```python
from build123d import *

# Parameters (mm, degrees)
BOSS_EXTRUDE1_DEPTH      = 6
BOSS_EXTRUDE2_DEPTH      = 40
CUT_EXTRUDE1_REACH       = 62.762
SKETCH9_R                = 1.6
CUT_EXTRUDE2_REACH       = 62.762
SKETCH10_R               = 7
BOSS_EXTRUDE4_DEPTH      = 25
BOSS_EXTRUDE5_REACH      = 73.576
SKETCH12_R               = 2.5
BOSS_EXTRUDE6_REACH      = 73.576
BOSS_EXTRUDE6_END_RADIUS = 23.21251372
SKETCH14_R               = 2.5
SKETCH17_W               = 26.966711831
SKETCH17_H               = 26.757667553
CUT_EXTRUDE4_DEPTH       = 6
FILLET1_R                = 2
SKETCH7_R                = 4
CUT_EXTRUDE5_DEPTH       = 3


with BuildPart() as part:
    # Sketch3 → Boss-Extrude1 (new body)
    with BuildSketch(Plane.XY):
        with BuildLine():
            Line((-20, 10.240601504), (20, 10.240601504))
            ThreePointArc((20, 10.240601504), (24.242640687, 8.483242191), (26, 4.240601504))
            Line((26, 4.240601504), (26, -13.759398496))
            ThreePointArc((26, -13.759398496), (24.242640687, -18.002039183), (20, -19.759398496))
            Line((20, -19.759398496), (-20, -19.759398496))
            ThreePointArc((-20, -19.759398496), (-24.242640687, -18.002039183), (-26, -13.759398496))
            Line((-26, -13.759398496), (-26, 4.240601504))
            ThreePointArc((-26, 4.240601504), (-24.242640687, 8.483242191), (-20, 10.240601504))
        make_face()
    extrude(amount=BOSS_EXTRUDE1_DEPTH)

    # Sketch4 → Boss-Extrude2 (add)
    with BuildSketch(Plane.XY.offset(6)):
        with BuildLine():
            Line((-26, 4.240601504), (26, 4.240601504))
            ThreePointArc((26, 4.240601504), (24.242640687, 8.483242191), (20, 10.240601504))
            Line((20, 10.240601504), (-20, 10.240601504))
            ThreePointArc((-20, 10.240601504), (-24.242640687, 8.483242191), (-26, 4.240601504))
        make_face()
    extrude(amount=BOSS_EXTRUDE2_DEPTH)

    # Sketch9 → Cut-Extrude1 (cut, up to next)
    with BuildSketch(Plane(origin=(0, 10.240601504, 0), x_dir=(1, 0, 0), z_dir=(0, 1, 0)), mode=Mode.PRIVATE) as cut_extrude1_sk1:
        with Locations(Location((0, -42.4, 0), (0, 0, 180))):
            Circle(SKETCH9_R)
    cut_extrude1_tool1 = extrude(cut_extrude1_sk1.sketch, amount=-CUT_EXTRUDE1_REACH, mode=Mode.PRIVATE) & part.part
    # Sketch9 → Cut-Extrude1 (cut, up to next)
    with BuildSketch(Plane(origin=(0, 10.240601504, 0), x_dir=(1, 0, 0), z_dir=(0, 1, 0)), mode=Mode.PRIVATE) as cut_extrude1_sk2:
        with Locations(Location((14.202816622, -34.2, 0), (0, 0, 180))):
            Circle(SKETCH9_R)
    cut_extrude1_tool2 = extrude(cut_extrude1_sk2.sketch, amount=-CUT_EXTRUDE1_REACH, mode=Mode.PRIVATE) & part.part
    # Sketch9 → Cut-Extrude1 (cut, up to next)
    with BuildSketch(Plane(origin=(0, 10.240601504, 0), x_dir=(1, 0, 0), z_dir=(0, 1, 0)), mode=Mode.PRIVATE) as cut_extrude1_sk3:
        with Locations(Location((-14.202816622, -34.2, 0), (0, 0, 180))):
            Circle(SKETCH9_R)
    cut_extrude1_tool3 = extrude(cut_extrude1_sk3.sketch, amount=-CUT_EXTRUDE1_REACH, mode=Mode.PRIVATE) & part.part
    # Sketch9 → Cut-Extrude1 (cut, up to next)
    with BuildSketch(Plane(origin=(0, 10.240601504, 0), x_dir=(1, 0, 0), z_dir=(0, 1, 0)), mode=Mode.PRIVATE) as cut_extrude1_sk4:
        with Locations(Location((-14.202816622, -17.8, 0), (0, 0, 180))):
            Circle(SKETCH9_R)
    cut_extrude1_tool4 = extrude(cut_extrude1_sk4.sketch, amount=-CUT_EXTRUDE1_REACH, mode=Mode.PRIVATE) & part.part
    # Sketch9 → Cut-Extrude1 (cut, up to next)
    with BuildSketch(Plane(origin=(0, 10.240601504, 0), x_dir=(1, 0, 0), z_dir=(0, 1, 0)), mode=Mode.PRIVATE) as cut_extrude1_sk5:
        with Locations(Location((0, -9.6, 0), (0, 0, 180))):
            Circle(SKETCH9_R)
    cut_extrude1_tool5 = extrude(cut_extrude1_sk5.sketch, amount=-CUT_EXTRUDE1_REACH, mode=Mode.PRIVATE) & part.part
    # Sketch9 → Cut-Extrude1 (cut, up to next)
    with BuildSketch(Plane(origin=(0, 10.240601504, 0), x_dir=(1, 0, 0), z_dir=(0, 1, 0)), mode=Mode.PRIVATE) as cut_extrude1_sk6:
        with Locations(Location((14.202816622, -17.8, 0), (0, 0, 180))):
            Circle(SKETCH9_R)
    cut_extrude1_tool6 = extrude(cut_extrude1_sk6.sketch, amount=-CUT_EXTRUDE1_REACH, mode=Mode.PRIVATE) & part.part
    add(cut_extrude1_tool1.solids().sort_by_distance((0, 10.240602, 42.4))[0], mode=Mode.SUBTRACT)
    add(cut_extrude1_tool2.solids().sort_by_distance((14.202817, 10.240602, 34.2))[0], mode=Mode.SUBTRACT)
    add(cut_extrude1_tool3.solids().sort_by_distance((-14.202817, 10.240602, 34.2))[0], mode=Mode.SUBTRACT)
    add(cut_extrude1_tool4.solids().sort_by_distance((-14.202817, 10.240602, 17.8))[0], mode=Mode.SUBTRACT)
    add(cut_extrude1_tool5.solids().sort_by_distance((0, 10.240602, 9.6))[0], mode=Mode.SUBTRACT)
    add(cut_extrude1_tool6.solids().sort_by_distance((14.202817, 10.240602, 17.8))[0], mode=Mode.SUBTRACT)

    # Sketch10 → Cut-Extrude2 (cut, up to next)
    with BuildSketch(Plane(origin=(0, 10.240601504, 0), x_dir=(1, 0, 0), z_dir=(0, 1, 0)), mode=Mode.PRIVATE) as cut_extrude2_sk1:
        with Locations(Location((-6.5, -26, 0), (0, 0, 180))):
            Circle(SKETCH10_R)
    cut_extrude2_tool1 = extrude(cut_extrude2_sk1.sketch, amount=-CUT_EXTRUDE2_REACH, mode=Mode.PRIVATE) & part.part
    add(cut_extrude2_tool1.solids().sort_by_distance((-6.5, 10.240602, 26))[0], mode=Mode.SUBTRACT)

    # Sketch11 → Boss-Extrude4 (add)
    with BuildSketch(Plane(origin=(0, 10.240601504, 0), x_dir=(1, 0, 0), z_dir=(0, 1, 0))):
        with BuildLine():
            Line((20, -14.217776389), (16.421656056, -16.443368147))
            ThreePointArc((16.421656056, -16.443368147), (0.037479345, -7.000036966), (-16.383825563, -16.378656023))
            Line((-16.383825563, -16.378656023), (-20, -14.217776389))
            ThreePointArc((-20, -14.217776389), (0, -2.78748628), (20, -14.217776389))
        make_face()
    extrude(amount=BOSS_EXTRUDE4_DEPTH)

    # Sketch12 → Boss-Extrude5 (add, up to next)
    with BuildSketch(Plane(origin=(7.879699248, -7.879699248, 0), x_dir=(0, 0, 1), z_dir=(-0.7071067811865489, 0.7071067811865462, 0)), mode=Mode.PRIVATE) as boss_extrude5_sk1:
        with Locations(Location((7.574761701, 20.594839086, 0), (0, 0, 90))):
            Circle(SKETCH12_R)
    boss_extrude5_tool1 = extrude(boss_extrude5_sk1.sketch, amount=BOSS_EXTRUDE5_REACH, mode=Mode.PRIVATE) - part.part
    add(boss_extrude5_tool1.solids().sort_by_distance((22.44245, 6.683051, 7.574762))[0])

    # Boss-Extrude6: up to this cylinder (the profile starts outside it)
    boss_extrude6_end = Plane(origin=(0, 6.81435, 26), z_dir=(0, -1, 0)) * Cylinder(BOSS_EXTRUDE6_END_RADIUS, 194.57702744, mode=Mode.PRIVATE)
    # Sketch14 → Boss-Extrude6 (add, up to the surface)
    with BuildSketch(Plane(origin=(-7.879699248, -7.879699248, 0), x_dir=(0, 0, -1), z_dir=(0.7071067811865487, 0.7071067811865465, 0)), mode=Mode.PRIVATE) as boss_extrude6_sk1:
        with Locations((-10.283332747, 20.780524406)):
            Circle(SKETCH14_R)
    boss_extrude6_tool1 = extrude(boss_extrude6_sk1.sketch, amount=BOSS_EXTRUDE6_REACH, mode=Mode.PRIVATE) - boss_extrude6_end
    add(boss_extrude6_tool1.solids().sort_by_distance((-22.573749, 6.81435, 10.283333))[0])

    # Sketch17 → Cut-Extrude4 (cut)
    with BuildSketch(Plane(origin=(0, 0, 0), x_dir=(-1, 0, 0), z_dir=(0, 0, -1))):
        with Locations((18.352928334, -9.138232272)):
            Rectangle(SKETCH17_W, SKETCH17_H)
    extrude(amount=-CUT_EXTRUDE4_DEPTH, mode=Mode.SUBTRACT)

    # Fillet1
    fillet1_edges = [part.edges().sort_by_distance(p)[0] for p in [
        (-4.869572418, -19.759398496, 3),
        (-4.869572418, 4.240601504, 3),
    ]]
    fillet(fillet1_edges, radius=FILLET1_R)

    # Sketch7 → Cut-Extrude5 (cut)
    with BuildSketch(Plane(origin=(0, 0, 0), x_dir=(-1, 0, 0), z_dir=(0, 0, -1))):
        with Locations((0, -4.759398496)):
            Circle(SKETCH7_R)
    extrude(amount=-CUT_EXTRUDE5_DEPTH, mode=Mode.SUBTRACT)


solid = part.part
```
Here's how the part is built. I have some questions about the finished solid (model axes, mm). A direction names the side the tool comes from. Coordinates: 2 decimals unless noted, no trailing zeros. Order: outer loops, then holes, each group sorted by start corner. A loop starts at its lowest first (then second) coordinate and runs counter-clockwise, first axis right, second up. Notation, with made-up numbers: (59, 79.25) - (91, 79.25) arc R33 ccw to (91, 110.25) - close; hole circle Ø9 at (20.25, 9.25). An arc over 180 degrees is marked (long way). One line per question, with ' | ' between items.
(1) Suppose I cut it at D-D on x = 6. List the corners of the cut face in (y, z) for me, and give its area (3 significant figures).
Report:
outline: (-19.76, 0) - (10.24, 0) - (10.24, 3.58) - (35.24, 3.58) - (35.24, 7.97) - (10.24, 7.97) - (10.24, 46) - (4.24, 46) - (4.24, 6) - (-19.76, 6) - close | area: 530 mm2
(2) If we mould it in two halves opening along Z, with no side actions, what happens to faces 1 (the flat face through (6, -1, 0)), 2 (the cylindrical face through (0.208, 7.283, 11.186)), 3 (the cylindrical face through (15.473, 7.283, 33.226)), 4 (the flat face through (-18.17, 22.57, 15.31))? For each: pulls with the +Z half, pulls with the -Z half, needs draft (parallel to the pull), parting line crosses it, or undercut.
Report:
face 1: pulls with the -Z half | face 2: undercut | face 3: undercut | face 4: pulls with the +Z half
(3) Will these pins go through, and if not, where does the flat tip stop? pin 1 (16 mm diameter, centred on x = -6.5, z = 26, fed in from +Y); pin 2 (4 mm diameter, centred on x = 6.5, y = 29, fed in from +Z); pin 3 (19 mm diameter, centred on x = 10, y = -2.5, fed in from +Z); pin 4 (3 mm diameter, centred on x = 13, y = 18.5, fed in from +Z).
Report:
pin 1: stops at y = 10.24 | pin 2: stops at z = 9.01 | pin 3: stops at z = 46 | pin 4: stops at z = 13.72
(4) For faces 5 (the flat face through (-4.87, -8, 3)), 6 (the cylindrical face through (0.521, -0.793, 1.479)), 7 (the flat face through (18.236, 22.566, 15.315)), 8 (the flat face through (0, 10.241, 31)), which set-ups out of +Z, -Z, +X, -X, +Y, -Y let a thin tool reach every point of the face, with its end or its side?
Report:
face 5: +Z, -Z, -X, -Y | face 6: -Z | face 7: +Z, +X, +Y | face 8: +Z, +Y
(5) Suppose I cut it at B-B on z = 17.8. List the corners of the cut face in (x, y) for me.
Report:
outline: (-26, 4.24) - (-15.8, 4.24) - (-15.8, 10.24) - (-20, 10.24) arc R6 ccw to start; (-12.6, 4.24) - (12.6, 4.24) - (12.6, 10.24) - (-12.6, 10.24) - close; (15.8, 4.24) - (26, 4.24) arc R6 ccw to (20, 10.24) - (15.8, 10.24) - close
(6) Suppose I cut it at A-A on z = 26. List the corners of the cut face in (x, y) for me, and give its area (3 significant figures).
Report:
outline: (-26, 4.24) - (-13.5, 4.24) - (-13.5, 10.24) - (-20, 10.24) arc R6 ccw to start; (0.5, 4.24) - (26, 4.24) arc R6 ccw to (20, 10.24) - (0.5, 10.24) - close | area: 213 mm2
(7) Suppose I cut it at C-C on y = 5. List the corners of the cut face in (x, z) for me.
Report:
outline: (-25.95, 0) - (25.95, 0) - (25.95, 46) - (-25.95, 46) - close; hole circle Ø3.2 at (-14.2, 17.8); hole circle Ø3.2 at (-14.2, 34.2); hole circle Ø14 at (-6.5, 26); hole circle Ø3.2 at (0, 9.6); hole circle Ø3.2 at (0, 42.4); hole circle Ø3.2 at (14.2, 17.8); hole circle Ø3.2 at (14.2, 34.2)
(8) If I drill on L1, parallel to Y at x = 10.5, z = 37; L2, parallel to Z at x = 1, y = -11; L3, parallel to X at y = 19, z = 9, over which ranges is the centre line in solid material (lowest first)?
Report:
L1: y = 4.24 to 10.24 | L2: z = 0 to 6 | L3: x = -15.81 to -8.49, 8.49 to 15.81
